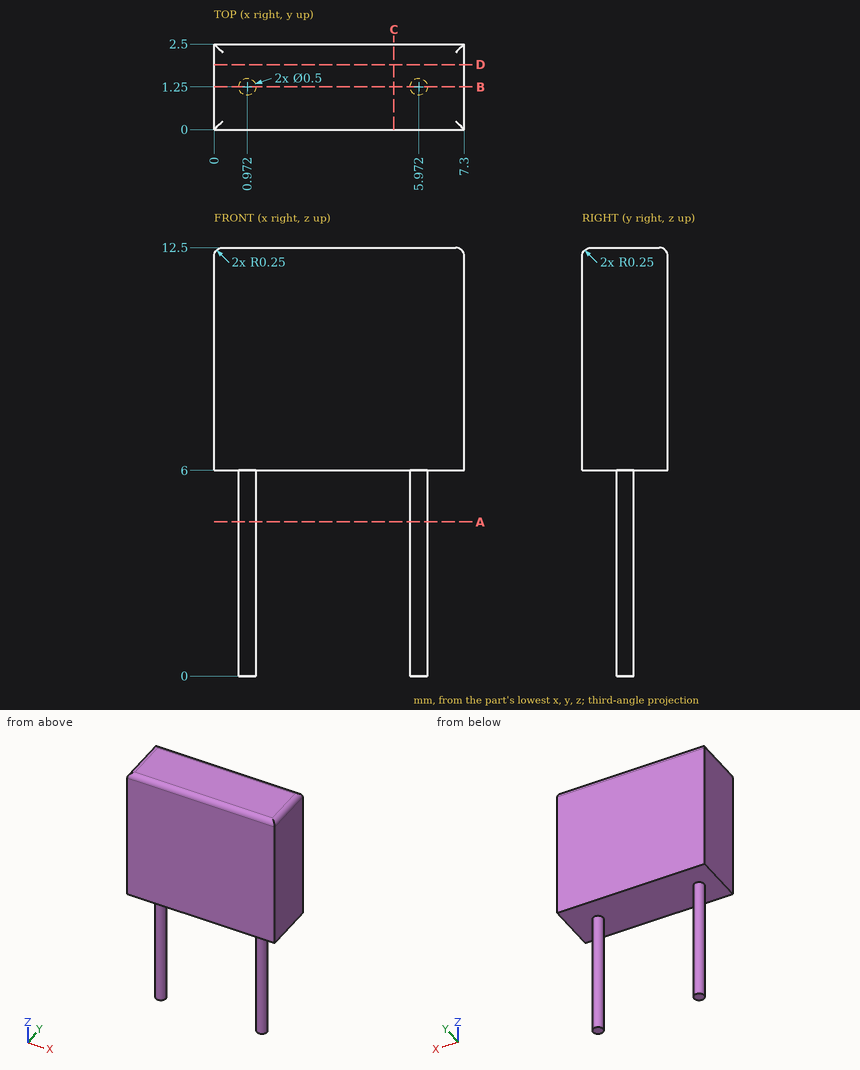
Here's the drawing with two shaded views (mm, measured from the low corner). I have some questions. Coordinates: 2 decimals unless noted, no trailing zeros. Loops run counter-clockwise (first coordinate to the right, second up) from the corner with the lowest first, then second, coordinate; pieces in that order, holes last. Notation, with made-up numbers: M 2,56 L 6,56 A37 ccw 6,94 Z; hole C -24.75,67.25 d10. An arc over 180 degrees is marked long. Put each result on its own line as item: value. Start each with the question number.
(1) Imagine slicing it at C-C on x = 5.25. List the corners of the cut face in (y, z) for me, and give its area (3 significant figures).
(2) I need wall thicknesses on probe 1 along Z at (x, y) = (3, 0.8). Which ranges of the line are inside material? Lowest first, please.
(3) Imagine slicing it at A-A on z = 4.5. List the corners of the cut face in (x, y) for me.
(4) Imagine slicing it at B-B on y = 1.25. List the corners of the cut face in (x, z) for me, and give its area (3 significant figures).
(5) Imagine slicing it at D-D on y = 1.9. List the corners of the cut face in (x, z) for me, and give its area (3 significant figures).
(6) Will this pin go through, and if not, where does the flat tip stop? pin 1 Ø0.8 at (x, y) = (4.5, 1) entering from -Z.
Worked answers:
1. outline: M 0,6 L 2.5,6 L 2.5,12.25 A0.25 ccw 2.25,12.5 L 0.25,12.5 A0.25 ccw 0,12.25 Z
1. area: 16.2 mm2
2. probe 1: z = 6 to 12.5
3. outline: C 0.97,1.25 d0.5; C 5.97,1.25 d0.5
4. outline: M 0,6 L 0.72,6 L 0.72,0 L 1.22,0 L 1.22,6 L 5.72,6 L 5.72,0 L 6.22,0 L 6.22,6 L 7.3,6 L 7.3,12.25 A0.25 ccw 7.05,12.5 L 0.25,12.5 A0.25 ccw 0,12.25 Z
4. area: 53.4 mm2
5. outline: M 0,6 L 7.3,6 L 7.3,12.25 A0.25 ccw 7.05,12.5 L 0.25,12.5 A0.25 ccw 0,12.25 Z
5. area: 47.4 mm2
6. pin 1: stops at z = 6
